Verification items for the finished model (mm, model axes). A direction names the side the tool comes from. Coordinates: 2 decimals unless noted, no trailing zeros. Loops run counter-clockwise (first coordinate to the right, second up) from the corner with the lowest first, then second, coordinate; pieces in that order, holes last. Notation, with made-up numbers: (-25.75, 58.5) - (-21.75, 58.5) arc R26 cw to (-21.75, 86.5) - close; hole circle Ø1 at (53.5, 32). An arc over 180 degrees is marked (long way). Answer as CSV lines item,"result". Start each with the question number.
1. Gauge pin test, flat ends, axial feed: P1, Ø6, axis at x = 12.5, y = 27, coming from the -Z side; P2, Ø9.5, axis at x = 8.5, y = 11, coming from the +Z side. Record the tip position at first contact, or that the pin passes through.
2. Release check for a two-part mould opening along X. For faces 4 (the flat face through (21, 15, 8)), 5 (the flat face through (20, 15, 9)), 6 (the cylindrical face through (0.49, 0.57, 15.4)) record: pulls with the +X half, pulls with the -X half, needs draft (parallel to the pull), parting line crosses it, or undercut.
3. Cross-section at D-D (y = 15). Enter the section's corners in (x, z), plus the area to 3 significant figures.
4. Cross-section at B-B (y = 4). Enter the section's corners in (x, z), plus the area to 3 significant figures.
5. Set-up check for faces 1 (the flat face through (1, 15, 8)), 2 (the cylindrical face through (9.96, 12.56, -0.99)), 3 (the cylindrical face through (13.726, 9.941, -3.972)): record each of +Z, -Z, +X, -X, +Y, -Y from which the full face is reachable in a straight line by a thin tool's end or side.
6. Cross-section at A-A (z = 4). Enter the section's corners in (x, y).
7. Cross-section at C-C (x = 10.5). Enter the section's corners in (y, z).
8. Material ranges on line 1 (Y direction, x = 10.5, z = 0.2); line 2 (X direction, y = 26.5, z = 4); line 3 (Z direction, x = 6.25, y = 14.5), recorded low to high. Write a range as [from, to].
```python
from build123d import *

# Parameters (mm, degrees)
F1_DEPTH = 30
F2_R     = 2.5
F3_DEPTH = 3
F4_R     = 6
F4_R_2   = 2.5
F5_DEPTH = 4
F6_R     = 2
F7_D     = 4
F7_DEPTH = 15
F7_TIP   = 1.2017212381


with BuildPart() as f1:
    # F0 (on Front) → F1 (new body)
    with BuildSketch(Plane.XZ):
        Polygon((0, 1), (0, 0), (21, 0), (21, 1), (21, 16), (20, 16), (20, 1), (1, 1), (1, 16), (0, 16), align=None)
    extrude(amount=-F1_DEPTH)

    # F2 (on face) → F3 (join)
    with BuildSketch(Plane.XY.offset(1)):
        with Locations((10.5, 15)):
            Circle(F2_R)
    extrude(amount=-F3_DEPTH)

    # F4 (on face) → F5 (join)
    with BuildSketch(Plane(origin=(0, 0, -2), x_dir=(1, 0, 0), z_dir=(0, 0, -1))):
        with Locations((10.5, -15)):
            Circle(F4_R)
        with Locations((10.5, -15)):
            Circle(F4_R_2, mode=Mode.SUBTRACT)
        with Locations((10.5, -15)):
            Circle(F4_R_2)
    extrude(amount=F5_DEPTH)

    # F6
    f6_edges = [f1.edges().sort_by_distance(p)[0] for p in [
        (20.5, 0, 16),
        (20.5, 30, 16),
        (0.5, 30, 16),
        (0.5, 0, 16),
    ]]
    fillet(f6_edges, radius=F6_R)

    # F7
    with Locations(Plane.XY.offset(1)):
        with Locations((10.5, 4), (10.5, 26)):
            Hole(F7_D / 2, depth=F7_DEPTH)
            with Locations((0, 0, -(F7_DEPTH + F7_TIP / 2))):  # 118° drill point
                Cone(0, F7_D / 2, F7_TIP, mode=Mode.SUBTRACT)


solid = f1.part
```
Values follow:
1,P1,"stops at z = 0"
1,P2,"stops at z = 1"
2,face 4,"pulls with the +X half"
2,face 5,"undercut"
2,face 6,"needs draft"
3,outline,"(0, 0) - (8, 0) - (8, -2) - (4.5, -2) - (4.5, -6) - (16.5, -6) - (16.5, -2) - (13, -2) - (13, 0) - (21, 0) - (21, 16) - (20, 16) - (20, 1) - (1, 1) - (1, 16) - (0, 16) - close"
3,area,"109 mm²"
4,outline,"(0, 0) - (8.5, 0) - (8.5, 1) - (1, 1) - (1, 16) - (0, 16) - close; (12.5, 0) - (21, 0) - (21, 16) - (20, 16) - (20, 1) - (12.5, 1) - close"
4,area,"47.0 mm²"
5,face 1,"+Z, +Y, -Y"
5,face 2,"none"
5,face 3,"-Z"
6,outline,"(0, 0) - (1, 0) - (1, 30) - (0, 30) - close; (20, 0) - (21, 0) - (21, 30) - (20, 30) - close"
7,outline,"(0, 0) - (2, 0) - (2, 1) - (0, 1) - close; (6, 0) - (12.5, 0) - (12.5, -2) - (9, -2) - (9, -6) - (21, -6) - (21, -2) - (17.5, -2) - (17.5, 0) - (24, 0) - (24, 1) - (6, 1) - close; (28, 0) - (30, 0) - (30, 1) - (28, 1) - close"
8,line 1,"y = [0, 2], [6, 24], [28, 30]"
8,line 2,"x = [0, 1], [20, 21]"
8,line 3,"z = [-6, -2], [0, 1]"
